from build123d import *

# Parameters (mm, degrees)
F0_R     = 4.7625
F1_DEPTH = 7.9375
F2_R     = 3.3147
F3_DEPTH = 2.921
F4_R     = 5.207
F5_DEPTH = 6.985
F6_SIZE2 = 1.9797340731
F6_SIZE  = 1.143
F7_R     = 2.38125
F8_DEPTH = 25.4
F8_TAPER = 5


with BuildPart() as f1:
    # F0 (on Top) → F1 (new body)
    with BuildSketch(Plane.XY):
        Circle(F0_R)
    extrude(amount=F1_DEPTH)

    # F2 (on face) → F3 (join)
    with BuildSketch(Plane.XY.offset(7.9375)):
        with BuildLine():
            Line((-14.9098, -9.525), (0, -9.525))
            ThreePointArc((0, -9.525), (9.525, 0), (0, 9.525))
            Line((0, 9.525), (-14.9098, 9.525))
            ThreePointArc((-14.9098, 9.525), (-24.4348, 0), (-14.9098, -9.525))
        make_face()
        with Locations((-16.51, 0)):
            Circle(F2_R, mode=Mode.SUBTRACT)
    extrude(amount=F3_DEPTH)

    # F4 (on face) → F5 (join)
    with BuildSketch(Plane.XY.offset(10.8585)):
        Circle(F4_R)
    extrude(amount=F5_DEPTH)

    # F6
    f6_edges = [f1.edges().sort_by_distance(p)[0] for p in [
        (-19.8247, 0, 10.8585),
    ]]
    f6_side = f1.faces().sort_by_distance((-19.8247, 0, 9.398))[0]
    chamfer(f6_edges, length=F6_SIZE, length2=F6_SIZE2, reference=f6_side)

    # F7 (on face) → F8 (cut)
    with BuildSketch(Plane(origin=(0, 0, 0), x_dir=(1, 0, 0), z_dir=(0, 0, -1))):
        Circle(F7_R)
    extrude(amount=-F8_DEPTH, taper=F8_TAPER, mode=Mode.SUBTRACT)


solid = f1.part
Model file for the job. Use its own axes, mm. A direction names the side the tool comes from. Give positions to 0.01 mm unless a question says otherwise; leave off trailing zeros. Loops run counter-clockwise (first coordinate to the right, second up) from the corner with the lowest first, then second, coordinate; pieces in that order, holes last.
1) Saw through at B-B (z = 8.5). Write the cut outline in (x, y) (3 decimals).
2) Saw through at C-C (y = 0). Count the separate pieces of the cut face and the enclosed holes in it, plus the area to 3 significant figures.
3) Wall check: line 1 (Z direction, x = -11, y = -5.5); line 2 (Y direction, x = -16.51, z = 8.6); line 3 (X direction, y = -1.25, z = 4.5). Give the ranges that are in metal, low to high.
4) Pull direction X, two halves, no side cores. Call faces 4 (the cylindrical face through (-19.82, 0.15, 8.81)), 5 (the cylindrical face through (-3.78, -2.9, 3.91)), 6 (the conical face through (-1.26, 0.97, 9.05)), 7 (the flat face through (-8, 0, 10.858)): +X half, -X half, draft (parallel to the pull), parting line (faces both ways), or undercut.
5) Saw through at A-A (x = -16.51). Write the cut outline in (y, z), plus the area to 3 significant figures.
6) Tool access for faces 1 (the cylindrical face through (4.967, 1.564, 14.302)), 2 (the flat face through (-8, 0, 7.938)), 3 (the flat face through (2, -2, 0)): list every direction of +Z, -Z, +X, -X, +Y, -Y with a clear straight run to the whole face (end or side of a thin tool).
7) Flat gauge pins, fed straight in: pin 1 Ø2 at (y, z) = (-4, 13) entering from -X; pin 2 Ø8 at (y, z) = (2.5, 7.5) entering from -X; pin 3 Ø5.5 at (x, y) = (-8.5, -4) entering from +Z; pin 4 Ø4 at (x, y) = (-16.51, 0) entering from +Z. Where does each tip first touch, or does it go through?
8) Saw through at D-D (x = -7.5). Write the cut outline in (y, z) (1 decimal).
Answer block:
1. outline: (-14.91, -9.525) - (0, -9.525) arc R9.525 ccw to (0, 9.525) - (-14.91, 9.525) arc R9.525 ccw to start; hole circle Ø6.629 at (-16.51, 0); hole circle Ø3.275 at (0, 0)
2. separate pieces: 3
2. enclosed holes: 0
2. area: 169 mm2
3. line 1: z = 7.94 to 10.86
3. line 2: y = -9.39 to -3.31, 3.31 to 9.39
3. line 3: x = -4.6 to -1.55, 1.55 to 4.6
4. face 4: undercut
4. face 5: parting line
4. face 6: undercut
4. face 7: draft
5. outline: (-9.39, 7.94) - (-3.31, 7.94) - (-3.31, 9.72) - (-5.29, 10.86) - (-9.39, 10.86) - close; (3.31, 7.94) - (9.39, 7.94) - (9.39, 10.86) - (5.29, 10.86) - (3.31, 9.72) - close
5. area: 33.2 mm2
6. face 1: +Z
6. face 2: -Z
6. face 3: -Z, +X, -X, +Y, -Y
7. pin 1: stops at x = -4.26
7. pin 2: stops at x = -24.43
7. pin 3: stops at z = 10.86
7. pin 4: passes through
8. outline: (-9.5, 7.9) - (9.5, 7.9) - (9.5, 10.9) - (-9.5, 10.9) - close
